```python
from build123d import *

# Parameters (mm, degrees)
BOSS_EXTRUDE1_DEPTH                            = 6.525
BOSS_EXTRUDE1_2_DEPTH                          = 6.525
BOSS_EXTRUDE1_3_DEPTH                          = 6.525
BOSS_EXTRUDE2_START                            = 6.525
BOSS_EXTRUDE2_DEPTH                            = 6
BOSS_EXTRUDE3_DEPTH                            = 4
FILLET1_R                                      = 10
FILLET2_R                                      = 3
CUT_EXTRUDE1_DEPTH                             = 1
CSK_FOR_M3_FLAT_HEAD_MACHINE_SCREW1_AT_2_COUNT = 2
CSK_FOR_M3_FLAT_HEAD_MACHINE_SCREW1_AT_2_PITCH = 16.585281374
CSK_FOR_M3_FLAT_HEAD_MACHINE_SCREW1_AT_3_COUNT = 2
CSK_FOR_M3_FLAT_HEAD_MACHINE_SCREW1_AT_3_PITCH = 41.156976568
CSK_FOR_M3_FLAT_HEAD_MACHINE_SCREW1_AT_4_COUNT = 2
CSK_FOR_M3_FLAT_HEAD_MACHINE_SCREW1_AT_4_PITCH = 53.622609719
CUT_EXTRUDE2_DEPTH                             = 4
FILLET3_R                                      = 5
MOVE_START                                     = -6.525
MOVE_FACE2_OUTLINE_R                           = 1.6
MOVE_FACE2_DEPTH                               = 0.125
MOVE_START_2                                   = 6.4
MOVE_FACE2_2_OUTLINE_R                         = 1.6
MOVE_FACE2_2_DEPTH                             = 0.125
MOVE_START_3                                   = -0.05
MOVE_FACE3_OUTLINE_W                           = 37.75
MOVE_FACE3_OUTLINE_H                           = 12.8
MOVE_FACE3_DEPTH                               = 12.8


with BuildPart() as part:
    # Sketch1 → Boss-Extrude1 (new body)
    with BuildSketch(Plane.XY):
        Polygon((25, 0), (-12.7, 0), (-36.405591591, -23.705591591), (-32.162950904, -27.948232278), (-10.214718626, -6), (25, -6), align=None)
    boss_extrude1 = extrude(amount=BOSS_EXTRUDE1_DEPTH)



with BuildPart() as body_2:
    # Sketch1 → Boss-Extrude1 2 (new body)
    with BuildSketch(Plane.XY):
        Polygon((-49.345645687, -10.765537495), (-21.061374439, 17.518733752), (-22.242640687, 18.7), (-31.900923472, 18.7), (-55.356053327, -4.755129855), align=None)
    boss_extrude1_2 = extrude(amount=BOSS_EXTRUDE1_2_DEPTH)


with BuildPart() as body_3:
    # Sketch1 → Boss-Extrude1 3 (new body)
    with BuildSketch(Plane.XY):
        Polygon((6, 18.7), (0, 12.7), (25, 12.7), (25, 18.7), align=None)
    boss_extrude1_3 = extrude(amount=BOSS_EXTRUDE1_3_DEPTH)


with BuildPart() as part_1:
    add(part.part)

    add(body_2.part)  # Boss-Extrude2 merges body 2

    add(body_3.part)  # Boss-Extrude2 merges body 3
    # Sketch1<3> → Boss-Extrude2 (add)
    with BuildSketch(Plane.XY.offset(BOSS_EXTRUDE2_START)):
        Polygon((-32.162950904, -27.948232278), (-10.214718626, -6), (25, -6), (25, 18.7), (-31.900923472, 18.7), (-55.356053327, -4.755129855), align=None)
    boss_extrude2 = extrude(amount=BOSS_EXTRUDE2_DEPTH)

    # Mirror2: Boss-Extrude1, Boss-Extrude1 2, Boss-Extrude1 3, Boss-Extrude2 across plane
    add(boss_extrude1.mirror(Plane.XY))
    add(boss_extrude1_2.mirror(Plane.XY))
    add(boss_extrude1_3.mirror(Plane.XY))
    add(boss_extrude2.mirror(Plane.XY))

    # Sketch2 → Boss-Extrude3 (add, symmetric)
    with BuildSketch(Plane.XY):
        Polygon((-32.162950904, -27.948232278), (3.051767722, -27.948232278), (25, -6), (-10.214718626, -6), align=None)
    extrude(amount=BOSS_EXTRUDE3_DEPTH, both=True)

    # Fillet1
    fillet1_edges = [part_1.edges().sort_by_distance(p)[0] for p in [
        (-31.900923472, 18.7, 0),
        (-10.214718626, -6, 8.2625),
        (-10.214718626, -6, -8.2625),
        (3.051767722, -27.948232278, 0),
    ]]
    fillet(fillet1_edges, radius=FILLET1_R)

    # Fillet2
    fillet2_edges = [part_1.edges().sort_by_distance(p)[0] for p in [
        (-22.653300859, -18.438582233, -12.525),
        (-22.653300859, -18.438582233, 12.525),
        (-45.092954493, 5.507968978, -12.525),
        (-45.092954493, 5.507968978, 12.525),
        (-31.585622172, 17.938795325, -12.525),
        (-31.585622172, 17.938795325, 12.525),
        (-9.899417326, -6.761204675, -12.525),
        (-9.899417326, -6.761204675, 12.525),
        (9.463708499, -6, 12.525),
        (-1.379393924, 18.7, 12.525),
        (-1.379393924, 18.7, -12.525),
        (9.463708499, -6, -12.525),
    ]]
    fillet(fillet2_edges, radius=FILLET2_R)

    # Sketch1<4> → Cut-Extrude1 (cut, symmetric)
    with BuildSketch(Plane.XY):
        Polygon((-49.345645687, -10.765537495), (-21.061374439, 17.518733752), (-22.242640687, 18.7), (-31.900923472, 18.7), (-55.356053327, -4.755129855), align=None)
    extrude(amount=CUT_EXTRUDE1_DEPTH, both=True, mode=Mode.SUBTRACT)

    # Sketch6 → CSK for M3 Flat Head Machine Screw1 (revolve, cut)
    with BuildSketch(Plane(origin=(-34.759502115, 9.831013716, 12.525), x_dir=(0, -1, 0), z_dir=(1, 0, 0))):
        Polygon((0, 0), (0, 25.05), (1.6, 25.05), (1.6, 5.55), (3.15, 4), (3.15, 0), align=None)
    csk_for_m3_flat_head_machine_screw1 = revolve(axis=Axis((-34.759502115, 9.831013716, 18.875), (0, 0, -1)), mode=Mode.SUBTRACT)

    # CSK for M3 Flat Head Machine Screw1 at 2: CSK for M3 Flat Head Machine Screw1 ×2
    with Locations(*[Vector(-0.7071067811865509, -0.7071067811865441, 0) * (i * CSK_FOR_M3_FLAT_HEAD_MACHINE_SCREW1_AT_2_PITCH) for i in range(1, CSK_FOR_M3_FLAT_HEAD_MACHINE_SCREW1_AT_2_COUNT)]):
        add(csk_for_m3_flat_head_machine_screw1, mode=Mode.SUBTRACT)

    # CSK for M3 Flat Head Machine Screw1 at 3: CSK for M3 Flat Head Machine Screw1 ×2
    with Locations(*[Vector(0.9964167811823362, -0.08457894642422821, 0) * (i * CSK_FOR_M3_FLAT_HEAD_MACHINE_SCREW1_AT_3_PITCH) for i in range(1, CSK_FOR_M3_FLAT_HEAD_MACHINE_SCREW1_AT_3_COUNT)]):
        add(csk_for_m3_flat_head_machine_screw1, mode=Mode.SUBTRACT)

    # CSK for M3 Flat Head Machine Screw1 at 4: CSK for M3 Flat Head Machine Screw1 ×2
    with Locations(*[Vector(0.9978906732683498, -0.06491690229855007, 0) * (i * CSK_FOR_M3_FLAT_HEAD_MACHINE_SCREW1_AT_4_PITCH) for i in range(1, CSK_FOR_M3_FLAT_HEAD_MACHINE_SCREW1_AT_4_COUNT)]):
        add(csk_for_m3_flat_head_machine_screw1, mode=Mode.SUBTRACT)

    # Sketch7 → Cut-Extrude2 (cut)
    with BuildSketch(Plane(origin=(0, 0, -12.525), x_dir=(-1, 0, 0), z_dir=(0, 0, -1))):
        Polygon((37.93826407, 10.682760415), (35.611248814, 13.00977567), (32.43248686, 12.158028972), (31.580740161, 8.979267018), (33.907755417, 6.652251762), (37.086517371, 7.503998461), align=None)
        Polygon((49.665828997, -1.044804513), (47.338813742, 1.282210743), (44.160051787, 0.430464044), (43.308305089, -2.74829791), (45.635320344, -5.075313166), (48.814082299, -4.223566467), align=None)
        Polygon((-15.459103466, 6.35), (-17.104551733, 9.2), (-20.395448267, 9.2), (-22.040896534, 6.35), (-20.395448267, 3.5), (-17.104551733, 3.5), align=None)
        Polygon((-2.959103466, 6.35), (-4.604551733, 9.2), (-7.895448267, 9.2), (-9.540896534, 6.35), (-7.895448267, 3.5), (-4.604551733, 3.5), align=None)
    extrude(amount=-CUT_EXTRUDE2_DEPTH, mode=Mode.SUBTRACT)

    # Fillet3
    fillet3_edges = [part_1.edges().sort_by_distance(p)[0] for p in [
        (-21.652007563, 18.109366876, -1),
        (-52.350849507, -7.760333675, 1),
        (-52.350849507, -7.760333675, -1),
        (-21.652007563, 18.109366876, 1),
    ]]
    fillet(fillet3_edges, radius=FILLET3_R)

    # Move Face2: read off the stored shape, not the designer's step
    # Move Face2 outline → Move Face2 (add)
    with BuildSketch(Plane.XY.offset(MOVE_START)):
        Polygon((-12.7, 0), (25, 0), (25, 12.7), (0, 12.7), align=None)
        with Locations((6.25, 6.35)):
            Circle(MOVE_FACE2_OUTLINE_R, mode=Mode.SUBTRACT)
        with Locations((18.75, 6.35)):
            Circle(MOVE_FACE2_OUTLINE_R, mode=Mode.SUBTRACT)
    extrude(amount=MOVE_FACE2_DEPTH)

    # Move Face2 2 outline → Move Face2 2 (add)
    with BuildSketch(Plane.XY.offset(MOVE_START_2)):
        Polygon((-12.7, 0), (25, 0), (25, 12.7), (0, 12.7), align=None)
        with Locations((6.25, 6.35)):
            Circle(MOVE_FACE2_2_OUTLINE_R, mode=Mode.SUBTRACT)
        with Locations((18.75, 6.35)):
            Circle(MOVE_FACE2_2_OUTLINE_R, mode=Mode.SUBTRACT)
    extrude(amount=MOVE_FACE2_2_DEPTH)

    # Move Face3: read off the stored shape, not the designer's step
    # Move Face3 outline → Move Face3 (cut)
    with BuildSketch(Plane(origin=(0, 0, 0), x_dir=(1, 0, 0), z_dir=(0, 1, 0)).offset(MOVE_START_3)):
        with Locations((6.125, 0)):
            Rectangle(MOVE_FACE3_OUTLINE_W, MOVE_FACE3_OUTLINE_H)
    extrude(amount=MOVE_FACE3_DEPTH, mode=Mode.SUBTRACT)


solid = part_1.part
```
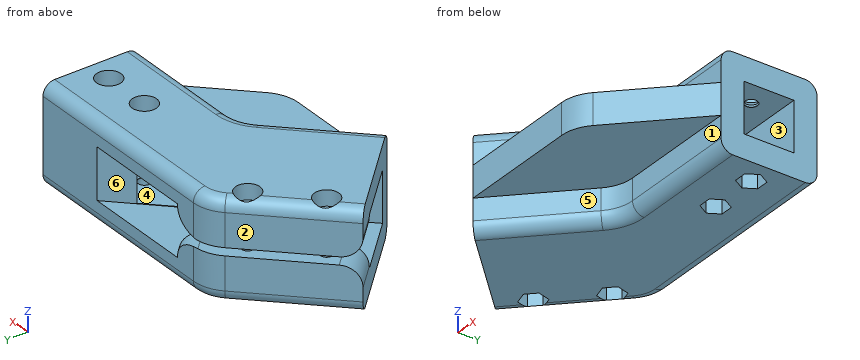
The listing builds one solid part. Answer for the finished solid, in the listing's coordinates (mm). Face numbers are marked on the shaded views. A direction names the side the tool comes from. Round coordinates to 2 decimals unless told otherwise and drop trailing zeros. Loops run counter-clockwise (first coordinate to the right, second up) from the corner with the lowest first, then second, coordinate; pieces in that order, holes last. Notation, with made-up numbers: (72.25, 9) - (102.25, 9) arc R7 ccw to (102.25, 16) - close; hole circle Ø7 at (79, -22.5). An arc over 180 degrees is marked (long way). Use one line per item in the form item = value. Start each with the question number.
1. The part is cut by section A-A on x = 12.5. Determine the outline of the cut face in (y, z) (3 decimals).
2. A tool of negligible diameter and unlimited length cuts with its end or side. For the marked faces 4, 5 and 6, from which of +Z, -Z, +X, -X, +Y, -Y can it reach the whole face along a straight path? Write none if from no direction.
3. Given pin 1 Ø6.5 at (x, y) = (5, 8.5) entering from +Z (3 decimals); pin 2 Ø5.5 at (x, y) = (6.25, 6.35) entering from -Z (3 decimals); pin 3 Ø12 at (x, z) = (-41.5, 3) entering from -Y; pin 4 Ø10 at (x, y) = (-1, -21) entering from -Z, each flat-ended and moving along its own axis, determine where each tip first touches the part or whether it passes through.
4. For a pull along Y with two mould halves and no side action, classify the marked faces 1, 2 and 3 as pulls with the +Y half, pulls with the -Y half, needs draft (parallel to the pull), parting line crosses it, or undercut.
5. Consider line 1 (Z direction, x = -28, y = 8) (3 decimals); line 2 (X direction, y = 6.35, z = -7.95); line 3 (Z direction, x = -10, y = 2) (3 decimals). Determine where each line is inside the solid, lowest interval first. Write a range as [from, to].
6. The part is cut by section B-B on x = -5. Determine the outline of the cut face in (y, z) (3 decimals).
Geometry check:
q1.outline = (-18.5, -4) - (-6, -4) - (-6, -9.525) arc R3 ccw to (-3, -12.525) - (15.7, -12.525) arc R3 ccw to (18.7, -9.525) - (18.7, 9.525) arc R3 ccw to (15.7, 12.525) - (-3, 12.525) arc R3 ccw to (-6, 9.525) - (-6, 4) - (-18.5, 4) - close; hole (-0.05, -6.4) - (12.75, -6.4) - (12.75, 6.4) - (-0.05, 6.4) - close
q2.face_4 = +X
q2.face_5 = -Z, +X, -Y
q2.face_6 = none
q3.pin_1 = 12.525
q3.pin_2 = -8.525
q3.pin_3 = -24.61
q3.pin_4 = -4
q4.face_1 = pulls with the -Y half
q4.face_2 = pulls with the +Y half
q4.face_3 = undercut
q5.line_1 = [-12.525, -6.525], [6.525, 12.525]
q5.line_2 = [-44.25, 4.65], [7.85, 17.15], [20.35, 25]
q5.line_3 = [-12.525, -6.4], [6.4, 12.525]
q6.outline = (-27.948, -4) - (-6, -4) - (-6, -9.525) arc R3 ccw to (-3, -12.525) - (15.7, -12.525) arc R3 ccw to (18.7, -9.525) - (18.7, -6.525) - (7.7, -6.525) - (7.7, -6.4) - (-0.05, -6.4) - (-0.05, 6.4) - (7.7, 6.4) - (7.7, 6.525) - (18.7, 6.525) - (18.7, 9.525) arc R3 ccw to (15.7, 12.525) - (-3, 12.525) arc R3 ccw to (-6, 9.525) - (-6, 4) - (-27.948, 4) - close
